Verification items for the finished model (mm, model axes). Face numbers are marked on the shaded views. Give positions to 0.01 mm unless a question says otherwise; leave off trailing zeros. Order: outer loops, then holes, each group sorted by start corner. A loop starts at its lowest first (then second) coordinate and runs counter-clockwise, first axis right, second up.
(1) Sectioned sample at B-B on x = 9. Record the cut outline in (y, z).
(2) Sectioned sample at C-C on z = 12. Record the cut outline in (x, y), plus the area to 3 significant figures.
(3) Scan lines: L1, parallel to X at y = -16, z = 9.5; L2, parallel to Y at x = -16.5, z = 14. Record each from-to range of solid material in increasing order.
(4) Gauge pin test, flat ends, axial feed: pin 1 (6 mm diameter, centred on y = 16, z = 21, fed in from +X); pin 2 (2 mm diameter, centred on x = -16.5, z = 20, fed in from +Y); pin 3 (1 mm diameter, centred on x = -13.5, z = 21, fed in from -Y). Record the tip position at first contact, or that the pin passes through.
(5) Sectioned sample at D-D on x = -19. Record the cut outline in (y, z).
(6) Mould release check, pull along Y, two halves, no side actions. Record for the marked faces 1, 2, 3 and 4: pulls with the +Y half, pulls with the -Y half, needs draft (parallel to the pull), parting line crosses it, or undercut.
(7) Sectioned sample at A-A on y = 0. Record the cut outline in (x, z).
```python
from build123d import *

# Parameters (mm, degrees)
F0_W     = 43
F0_H     = 43
F0_R     = 1.75
F0_R_2   = 15
F1_DEPTH = 30
F2_SIZE  = 8
F3_R     = 2


with BuildPart() as f1:
    # F0 (on Top) → F1 (new body)
    with BuildSketch(Plane.XY):
        Rectangle(F0_W, F0_H)
        with Locations((-15.5, -15.5)):
            Circle(F0_R, mode=Mode.SUBTRACT)
        with Locations((15.5, -15.5)):
            Circle(F0_R, mode=Mode.SUBTRACT)
        with Locations((-15.5, 15.5)):
            Circle(F0_R, mode=Mode.SUBTRACT)
        Circle(F0_R_2, mode=Mode.SUBTRACT)
        with Locations((15.5, 15.5)):
            Circle(F0_R, mode=Mode.SUBTRACT)
    extrude(amount=F1_DEPTH)

    # F2
    f2_edges = [f1.edges().sort_by_distance(p)[0] for p in [
        (-21.5, -21.5, 15),
        (21.5, -21.5, 15),
        (21.5, 21.5, 15),
        (-21.5, 21.5, 15),
    ]]
    chamfer(f2_edges, length=F2_SIZE)

    # F3
    f3_edges = [f1.edges().sort_by_distance(p)[0] for p in [
        (-13.5, 21.5, 15),
        (13.5, 21.5, 15),
        (21.5, 13.5, 15),
        (-21.5, 13.5, 15),
        (21.5, -13.5, 15),
        (13.5, -21.5, 15),
        (-13.5, -21.5, 15),
        (-21.5, -13.5, 15),
    ]]
    fillet(f3_edges, radius=F3_R)


solid = f1.part
```
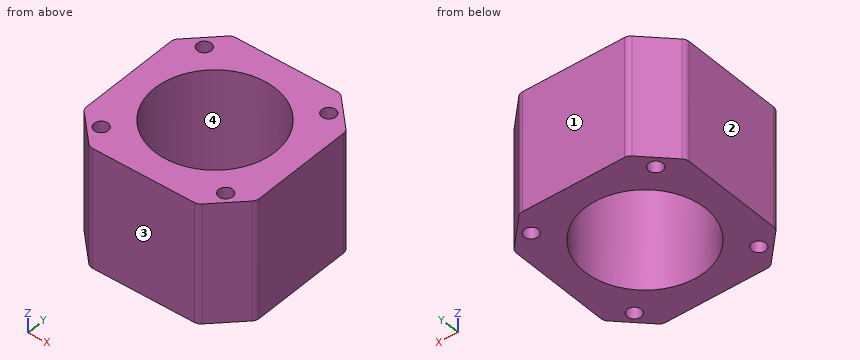
Ans:
1. outline: (-21.5, 0) - (-12, 0) - (-12, 30) - (-21.5, 30) - close; (12, 0) - (21.5, 0) - (21.5, 30) - (12, 30) - close
2. outline: (-21.5, -12.67) arc R2 ccw to (-20.91, -14.09) - (-14.09, -20.91) arc R2 ccw to (-12.67, -21.5) - (12.67, -21.5) arc R2 ccw to (14.09, -20.91) - (20.91, -14.09) arc R2 ccw to (21.5, -12.67) - (21.5, 12.67) arc R2 ccw to (20.91, 14.09) - (14.09, 20.91) arc R2 ccw to (12.67, 21.5) - (-12.67, 21.5) arc R2 ccw to (-14.09, 20.91) - (-20.91, 14.09) arc R2 ccw to (-21.5, 12.67) - close; hole circle Ø3.5 at (-15.5, -15.5); hole circle Ø3.5 at (-15.5, 15.5); hole circle Ø30 at (0, 0); hole circle Ø3.5 at (15.5, -15.5); hole circle Ø3.5 at (15.5, 15.5)
2. area: 975 mm2
3. L1: x = -19 to -17.18, -13.82 to 13.82, 17.18 to 19
3. L2: y = -18.5 to -16.94, -14.06 to 14.06, 16.94 to 18.5
4. pin 1: stops at x = 21.47
4. pin 2: stops at y = 19.5
4. pin 3: stops at y = -21.47
5. outline: (-16, 0) - (16, 0) - (16, 30) - (-16, 30) - close
6. face 1: pulls with the +Y half
6. face 2: needs draft
6. face 3: pulls with the -Y half
6. face 4: undercut
7. outline: (-21.5, 0) - (-15, 0) - (-15, 30) - (-21.5, 30) - close; (15, 0) - (21.5, 0) - (21.5, 30) - (15, 30) - close
